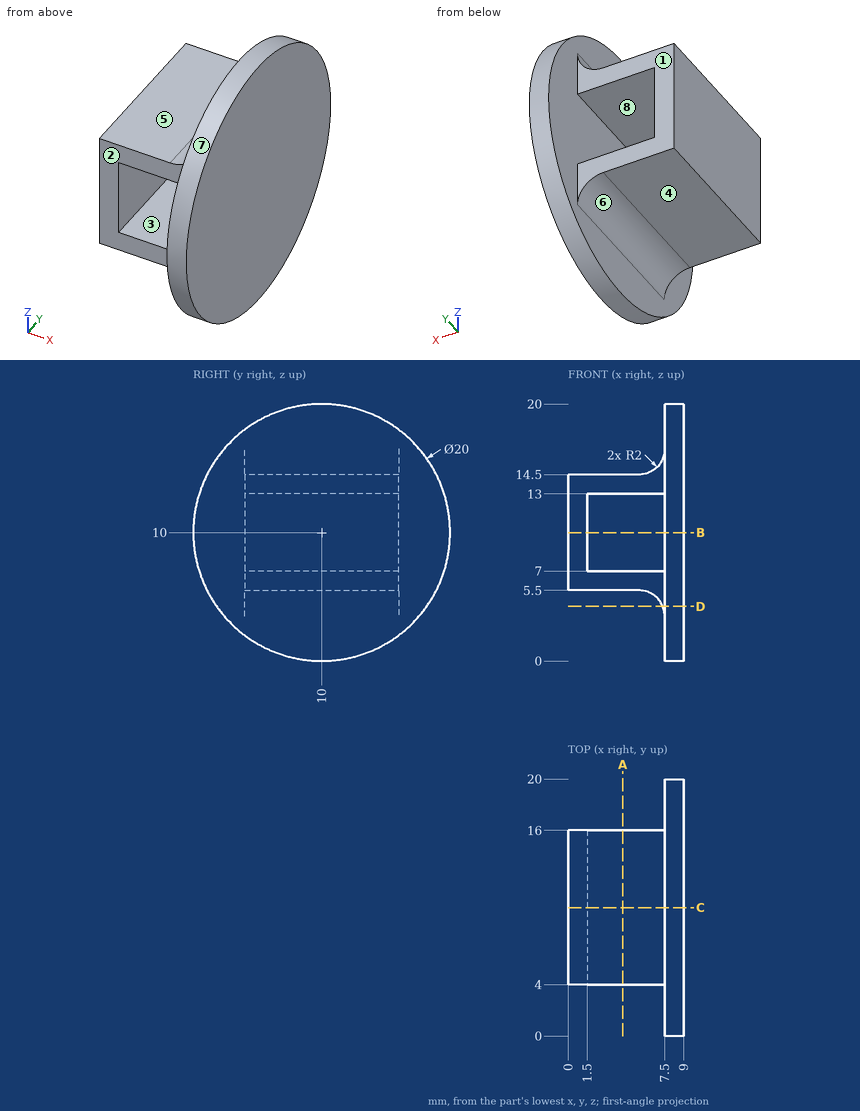
Verification items for this drawing (mm, ordinates from the low corner). A direction names the side the tool comes from. Give positions to 0.01 mm unless a question says otherwise; leave off trailing zeros. Loops run counter-clockwise (first coordinate to the right, second up) from the corner with the lowest first, then second, coordinate; pieces in that order, holes last. Notation, with made-up numbers: M 3,-4 L 46,-4 A25 cw 46,26 Z; hole C -5,12 d8. An arc over 180 degrees is marked long. Answer as CSV lines item,"result".
Item 1: Cross-section at B-B on z = 10. Record the cut outline in (x, y), and give its area (3 significant figures).
Values:
outline,"M 0,4 L 1.5,4 L 1.5,16 L 0,16 Z; M 7.5,0 L 9,0 L 9,20 L 7.5,20 Z"
area,"48.0 mm²"
Item 2: Access from +Z, -Z, +X, -X, +Y, -Y to the whole of each face (thin tool, end or side, straight path). Record for the marked faces 1, 2, 3, 4 and 5.
Values:
face 1,"+Z, -Z, -X, +Y"
face 2,"+Z, -Z, -X, -Y"
face 3,"+Y, -Y"
face 4,"-Z, -X, +Y, -Y"
face 5,"+Z, -X, +Y, -Y"
Item 3: Cross-section at C-C on y = 10. Record the cut outline in (x, z), and give its area (3 significant figures).
Values:
outline,"M 0,5.5 L 5.5,5.5 A2 cw 7.5,3.5 L 7.5,0 L 9,0 L 9,20 L 7.5,20 L 7.5,16.5 A2 cw 5.5,14.5 L 0,14.5 Z; hole M 1.5,7 L 7.5,7 L 7.5,13 L 1.5,13 Z"
area,"63.2 mm²"
Item 4: Depth check by flat-ended pin: P1, Ø1.5, axis at x = 3.5, z = 5.5, coming from the +Y side; P2, Ø4.5, axis at x = 2.5, y = 11, coming from the +Z side; P3, Ø3, axis at x = 1, y = 10, coming from the -Z side; P4, Ø5, axis at y = 15, z = 4.5, coming from the -X side. Enter the tip coordinate at first touch or a pass-through.
Values:
P1,"stops at y = 16"
P2,"stops at z = 14.5"
P3,"stops at z = 5.5"
P4,"stops at x = 0"
Item 5: Material ranges on line 1 (X direction, y = 13.75, z = 12); line 2 (Z direction, x = 3.5, y = 9); line 3 (X direction, y = 16.5, z = 5), recorded low to high.
Values:
line 1,"x = 0 to 1.5, 7.5 to 9"
line 2,"z = 5.5 to 7, 13 to 14.5"
line 3,"x = 7.5 to 9"
Item 6: Cross-section at A-A on x = 4.25. Record the cut outline in (y, z), and give its area (3 significant figures).
Values:
outline,"M 4,5.5 L 16,5.5 L 16,7 L 4,7 Z; M 4,13 L 16,13 L 16,14.5 L 4,14.5 Z"
area,"36.0 mm²"
Item 7: Cross-section at D-D on z = 4.25. Record the cut outline in (x, y), and give its area (3 significant figures).
Values:
outline,"M 7.35,4 L 7.5,4 L 7.5,1.82 L 9,1.82 L 9,18.18 L 7.5,18.18 L 7.5,16 L 7.35,16 Z"
area,"26.3 mm²"
Item 8: Release check for a two-part mould opening along Z. For the marked faces 6, 7 and 8 record: pulls with the +Z half, pulls with the -Z half, needs draft (parallel to the pull), parting line crosses it, or undercut.
Values:
face 6,"pulls with the -Z half"
face 7,"parting line crosses it"
face 8,"undercut"
